Verification items for the finished model (mm, model axes). A direction names the side the tool comes from. Coordinates: 2 decimals unless noted, no trailing zeros. Loops run counter-clockwise (first coordinate to the right, second up) from the corner with the lowest first, then second, coordinate; pieces in that order, holes last. Notation, with made-up numbers: (77, 79) -> (90, 79) arc R9 cw to (90, 95) -> close; hole circle Ø10 at (72, -22). An arc over 180 degrees is marked (long way). Write item = value, one per line.
```python
from build123d import *

# Parameters (mm, degrees)
F4_R = 1


# Not quite as in the source:
# - a fillet or chamfer that OpenCascade refuses, or shapes differently, is made with other operations: its cross-section is extruded or revolved along the edge and cut away or added


with BuildPart() as f1:
    # F0 (on Front) → F1 (revolve)
    with BuildSketch(Plane.XZ):
        with BuildLine():
            Line((0, 12), (0, 10))
            Line((0, 10), (3.1, 10))
            Line((3.1, 10), (3.1, 0))
            Line((3.1, 0), (8.5, 0))
            ThreePointArc((8.5, 0), (7.2147663015, 6.4382422656), (7, 13))
            Line((7, 13), (5, 13))
            Line((5, 13), (4, 12))
            Line((4, 12), (0, 12))
        make_face()
    revolve(axis=Axis((0, 0, 11), (0, 0, -1)))

    # F3: chamfer of 0.8 on 2 edges, made by hand

    # F3_s1 → F3_t2 (revolve, cut)
    with BuildSketch(Plane.XZ):
        Polygon((3.1, 0.8), (3.9, 0), (3.1, 0), align=None)
    revolve(axis=Axis((0, 0, 0), (0, 0, -1)), mode=Mode.SUBTRACT)

    # F3_s3 → F3_t4 (revolve, cut)
    with BuildSketch(Plane.XZ):
        with BuildLine():
            Line((7.4526927913, 0), (8.2271718294, 1.0004550311))
            ThreePointArc((8.2271718294, 1.0004550311), (8.3578103434, 0.5086375801), (8.5, 0))
            Line((8.5, 0), (7.4526927913, 0))
        make_face()
    revolve(axis=Axis((0, 0, 0), (0, 0, -1)), mode=Mode.SUBTRACT)

    # F4
    f4_edges = [f1.edges().sort_by_distance(p)[0] for p in [
        (-7, 0, 13),
    ]]
    fillet(f4_edges, radius=F4_R)


solid = f1.part
```
1) Release check for a two-part mould opening along X. For faces 3 (the face through (-3, 3, 0)), 4 (the face through (1.43, 2.75, 5.34)), 5 (the face through (0, 0, 10)) record: pulls with the +X half, pulls with the -X half, needs draft (parallel to the pull), parting line crosses it, or undercut.
Ans:
face_3 = needs draft
face_4 = undercut
face_5 = undercut
2) Material ranges on line 1 (Y direction, x = -1.25, z = 3.25); line 2 (X direction, y = 0, z = 2.5); line 3 (Z direction, x = 0.5, y = 1), recorded low to high.
Ans:
line_1 = -7.61 to -2.84, 2.84 to 7.61
line_2 = -7.87 to -3.1, 3.1 to 7.87
line_3 = 10 to 12
3) Depth check by flat-ended pin: pin 1 Ø4 at (x, z) = (-0.5, 6) entering from +Y; pin 2 Ø5 at (x, y) = (-0.5, -0.5) entering from -Z; pin 3 Ø4 at (x, y) = (6, -4) entering from -Z; pin 4 Ø3.5 at (x, y) = (0, 0) entering from -Z. Enter the tip coordinate at first touch or a pass-through.
Ans:
pin_1 = 7.57
pin_2 = 0.69
pin_3 = 0
pin_4 = 10
4) Sectioned sample at A-A, the plane z = 8.75. Record the cut outline in (x, y).
Ans:
outline = circle Ø14.03 at (0, 0); hole circle Ø6.2 at (0, 0)
5) Tool access check on faces 1 (the face through (-4, 4, 13)), 2 (the face through (0, 0, 12)). Record the directions out of +Z, -Z, +X, -X, +Y, -Y that give a thin tool (end or side, any length) a straight path to the whole face; none if there is none.
Ans:
face_1 = +Z, +X, -X, +Y, -Y
face_2 = +Z
6) Sectioned sample at B-B, the plane z = 6.75. Record the cut outline in (x, y).
Ans:
outline = circle Ø14.36 at (0, 0); hole circle Ø6.2 at (0, 0)
